Check sheet for the modelled part. Datum: model origin and axes. Units: mm. Face numbers are marked on the shaded views. Give positions to 0.01 mm unless a question says otherwise; leave off trailing zeros. Order: outer loops, then holes, each group sorted by start corner. A loop starts at its lowest first (then second) coordinate and runs counter-clockwise, first axis right, second up.
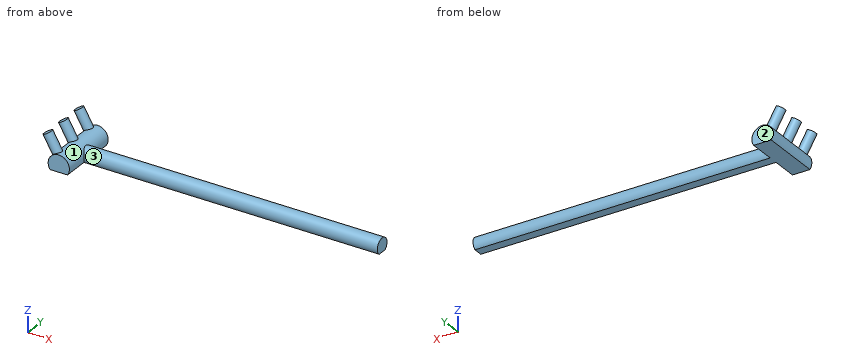
```python
from build123d import *

# Parameters (mm, degrees)
F1_DEPTH        = 10
F3_DEPTH        = 100
F5_R            = 1.5
F6_DEPTH        = 10
F6_COPIES_COUNT = 2
F6_COPIES_PITCH = 8


# Not quite as in the source:
# - a pattern or mirror of a feature is missing from the dataset's text; its kind, count and spacing are read off the source's solid


with BuildPart() as f1:
    # F0 (on Front) → F1 (new body, symmetric)
    with BuildSketch(Plane.XZ):
        with BuildLine():
            Line((-2.8722813233, -2), (2.8722813233, -2))
            ThreePointArc((2.8722813233, -2), (0, 3.5), (-2.8722813233, -2))
        make_face()
    extrude(amount=F1_DEPTH, both=True)

    # F2 (on Right) → F3 (join)
    with BuildSketch(Plane.YZ):
        with BuildLine():
            Line((-1.5, -2), (1.5, -2))
            ThreePointArc((1.5, -2), (0, 2.5), (-1.5, -2))
        make_face()
    extrude(amount=F3_DEPTH)

    # F5 (on face) → F6 (join)
    with BuildSketch(Plane(origin=(0.147955073, 0, -0.2562657036), x_dir=(0.8660254038, 0, 0.5), z_dir=(0.5, 0, -0.8660254038))):
        Circle(F5_R)
        with Locations((0, -8)):
            Circle(F5_R)
    f6 = extrude(amount=-F6_DEPTH)

    # F6_copies: F6 ×2
    with Locations(*[(0, -i * F6_COPIES_PITCH, 0) for i in range(1, F6_COPIES_COUNT)]):
        add(f6)


solid = f1.part
```
(1) Cross-section at D-D on z = 6. Count the separate pieces of the cut face and the enclosed holes in it, then the cut area to 3 significant figures.
Response values:
separate pieces: 3
enclosed holes: 0
area: 24.5 mm2
(2) Material ranges on L1, parallel to Z at x = 64, y = 0.5; L2, parallel to Y at x = 83, z = 2; L3, parallel to X at y = 2.25, z = 0, recorded low to high.
Response values:
L1: z = -2 to 2.45
L2: y = -1.5 to 1.5
L3: x = -3.5 to 100
(3) Cross-section at C-C on y = 0. Enter the section's corners in (x, z), then the cut area to 3 significant figures.
Response values:
outline: (-6.15, 7.65) - (-2.88, 1.99) arc R3.5 ccw to (-2.87, -2) - (100, -2) - (100, 2.5) - (2.45, 2.5) arc R3.5 ccw to (-0.28, 3.49) - (-3.55, 9.15) - close
area: 487 mm2
(4) Cross-section at A-A on z = 0. Enter the section's corners in (x, y), then the cut area to 4 significant figures.
Response values:
outline: (-3.5, -10) - (3.5, -10) - (3.5, -2.5) - (100, -2.5) - (100, 2.5) - (3.5, 2.5) - (3.5, 10) - (-3.5, 10) - close
area: 622.5 mm2
(5) Release check for a two-part mould opening along Y. For the marked faces 1, 2 and 3 record: released by +Y, released by -Y, zero draft, split by the parting line, or undercut.
Response values:
face 1: undercut
face 2: released by +Y
face 3: split by the parting line
(6) Gauge pin test, flat ends, axial feed: pin 1 Ø6 at (x, y) = (11.5, -5) entering from -Z; pin 2 Ø1.5 at (y, z) = (-2, 2.5) entering from -X; pin 3 Ø1 at (y, z) = (-6.5, 7) entering from -X. Record the tip position at first contact, or that the pin passes through.
Response values:
pin 1: stops at z = -1.5
pin 2: stops at x = -3.03
pin 3: stops at x = -5.4
(7) Cross-section at B-B on x = 6. Enter the section's corners in (y, z), then the cut area to 3 significant figures.
Response values:
outline: (-1.5, -2) - (1.5, -2) arc R2.5 ccw (long way) to start
area: 18.6 mm2
